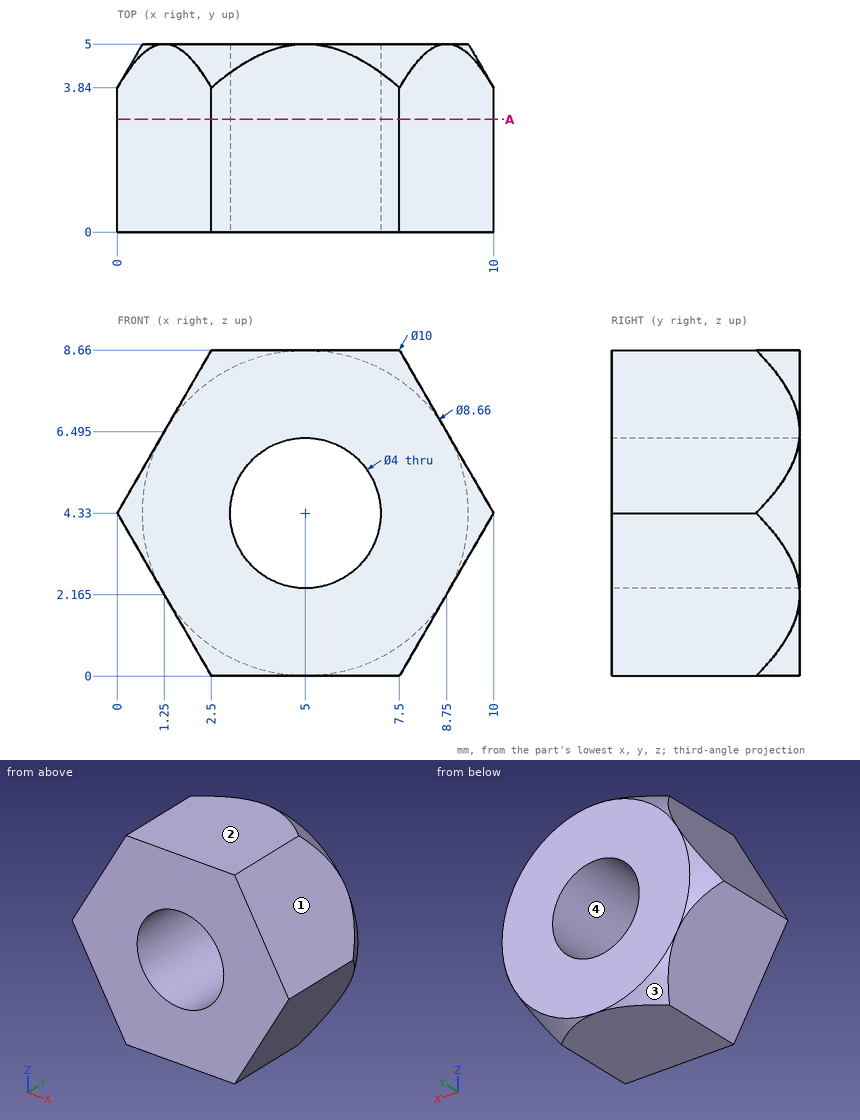
Study the drawing (mm; zero at the part's minimum x, y, z) and answer. Round coordinates to 2 decimals unless told otherwise and drop trailing zeros. Order: outer loops, then holes, each group sorted by start corner. A loop starts at its lowest first (then second) coordinate and runs counter-clockwise, first axis right, second up. Notation, with made-up numbers: (72, 10.5) - (111, 10.5) arc R16 cw to (111, 19.5) - close; hole circle Ø8 at (38.5, -19). An arc over 180 degrees is marked (long way). Use one line per item in the form item = value. Start each with the question number.
(1) The part is cut by section A-A (y = 3). Give the vertices of the cut face in (x, z).
(2) Flat-ended cylindrical pins translate along their axes: pin 1 Ø3 at (y, z) = (4, 1.5) entering from -X; pin 2 Ø1.5 at (y, z) = (2, 7.5) entering from +X. Find the tip coordinate at first contact, or state that the pin passes through.
(3) Determine the mould class of the marked faces 1, 2, 3 and 4 for opening direction X: +X half, -X half, draft (parallel to the pull), parting line (faces both ways), or undercut.
(4) Find the intervals of material crossed by line 1 along X through (y, z) = (3.75, 6.5); line 2 along X through (y, z) = (2.75, 4.5); line 3 along X through (y, z) = (0.3, 5.75), in increasing order. Write a range as from..to.
Checked values:
q1.outline = (0, 4.33) - (2.5, 0) - (7.5, 0) - (10, 4.33) - (7.5, 8.66) - (2.5, 8.66) - close; hole circle Ø4 at (5, 4.33)
q2.pin_1 = 0.77
q2.pin_2 = 8.6
q3.face_1 = +X half
q3.face_2 = draft
q3.face_3 = -X half
q3.face_4 = undercut
q4.line_1 = 1.25..8.75
q4.line_2 = 0.1..3.01, 6.99..9.9
q4.line_3 = 0.82..3.59, 6.41..9.18
